The figure shows three views and two pictorial views of one solid part (mm, origin at its lowest corner). Answer the questions. Give positions to 0.01 mm unless a question says otherwise; leave off trailing zeros. Loops run counter-clockwise (first coordinate to the right, second up) from the corner with the lowest first, then second, coordinate; pieces in that order, holes last. Notation, with made-up numbers: (87.5, 75) - (127.5, 75) arc R8 cw to (127.5, 90) - close; hole circle Ø3 at (-21, -21.5). An arc over 180 degrees is marked (long way). Write item = value, one per line.
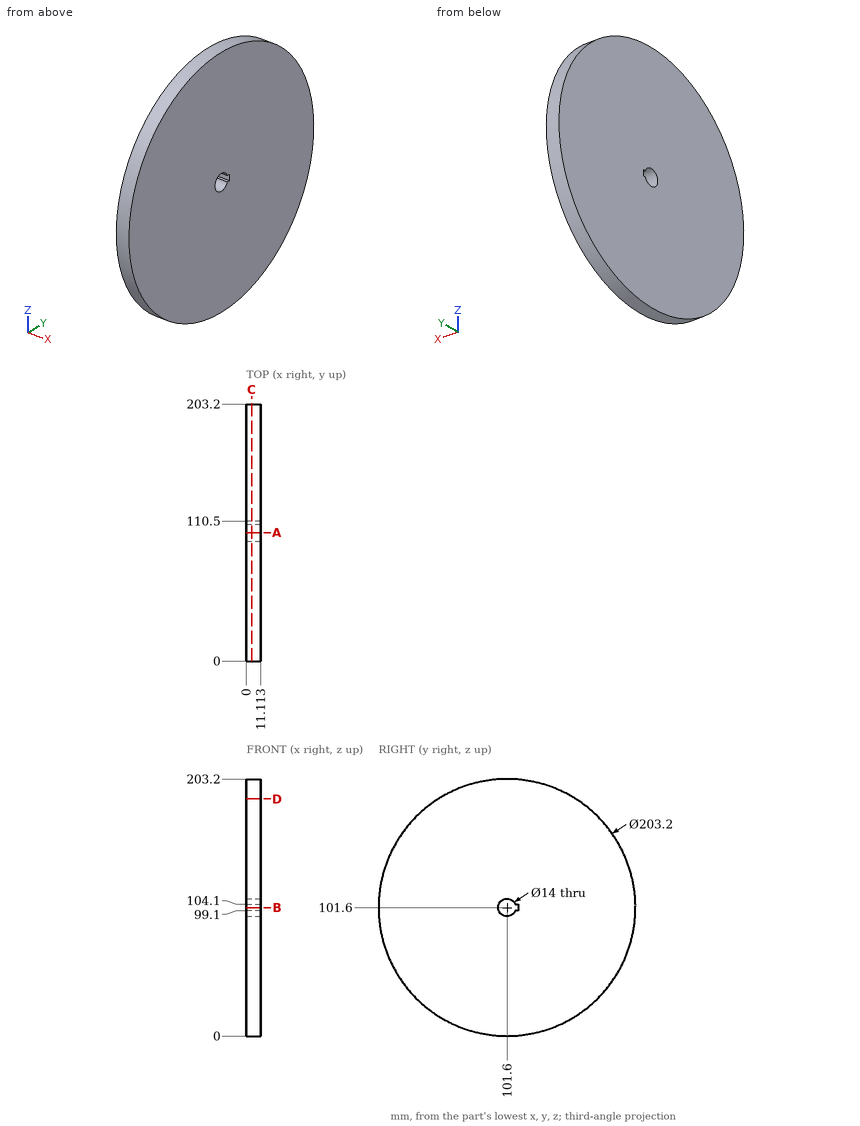
1) A cutting plane is placed at D-D on z = 187.5. Determine the outline of the cut face in (x, y), then the cut area to 3 significant figures.
Output:
outline = (0, 47.34) - (11.11, 47.34) - (11.11, 155.86) - (0, 155.86) - close
area = 1,210 mm²
2) A cutting plane is placed at A-A on y = 101.6. Determine the outline of the cut face in (x, z), then the cut area to 3 significant figures.
Output:
outline = (0, 0) - (11.11, 0) - (11.11, 94.6) - (0, 94.6) - close; (0, 108.6) - (11.11, 108.6) - (11.11, 203.2) - (0, 203.2) - close
area = 2,100 mm²
3) Find the intervals of material crossed by probe 1 along Z at (x, y) = (8.5, 100.5) (1 decimal); probe 2 along Y at (x, z) = (5.5, 142); probe 3 along Y at (x, z) = (1.5, 84) (1 decimal), in increasing order.
Output:
probe_1 = 0 to 94.7, 108.5 to 203.2
probe_2 = 8.38 to 194.82
probe_3 = 1.5 to 201.7
4) A cutting plane is placed at B-B on z = 101.6. Determine the outline of the cut face in (x, y).
Output:
outline = (0, 0) - (11.11, 0) - (11.11, 94.6) - (0, 94.6) - close; (0, 110.5) - (11.11, 110.5) - (11.11, 203.2) - (0, 203.2) - close
5) Each of these flat-tipped pins is pushed along its axis until it touches: P1, Ø1, axis at y = 175.5, z = 65, coming from the -X side; P2, Ø5, axis at x = 1, y = 72.5, coming from the +Z side; P3, Ø3, axis at x = 4, z = 47.5, coming from the +Y side (1 decimal); P4, Ø5, axis at x = 6, y = 21.5, coming from the +Z side. Where does it stop, or does it pass through?
Output:
P1 = 0
P2 = 199.66
P3 = 188.5
P4 = 167.18
6) A cutting plane is placed at C-C on x = 4. Determine the outline of the cut face in (y, z), then the cut area to 3 significant figures.
Output:
outline = circle Ø203.2 at (101.6, 101.6); hole (108.14, 99.1) - (110.5, 99.1) - (110.5, 104.1) - (108.14, 104.1) arc R7 ccw (long way) to start
area = 32,300 mm²
